```python
from build123d import *

# Parameters (mm, degrees)
F0_R      = 14.3002
F1_DEPTH  = 40.5892
F2_W      = 11.867738
F2_H      = 43.622876
F2_W_2    = 10.350018
F3_DEPTH  = 37.084
F5_R      = 18.288
F6_DEPTH  = 1.651
F7_W      = 12.7
F7_H      = 5.3975
F8_DEPTH  = 9.7536
F9_W      = 0.7874
F9_H      = 7.62
F9_W_2    = 0.8128
F10_DEPTH = 9.5631


with BuildPart() as f1:
    # F0 (on Front) → F1 (new body)
    with BuildSketch(Plane.XZ):
        Circle(F0_R)
    extrude(amount=-F1_DEPTH)

    # F2 (on face) → F3 (cut)
    with BuildSketch(Plane.XZ):
        with Locations((-19.027569, 0.496973)):
            Rectangle(F2_W, F2_H)
        with Locations((18.268709, 0.496973)):
            Rectangle(F2_W_2, F2_H)
    extrude(amount=-F3_DEPTH, mode=Mode.SUBTRACT)

    # F5 (on offset) → F6 (join)
    with BuildSketch(Plane(origin=(0, 38.6842, 0), x_dir=(1, 0, 0), z_dir=(0, 1, 0))):
        Circle(F5_R)
    extrude(amount=-F6_DEPTH)

    # F7 (on face) → F8 (cut)
    with BuildSketch(Plane(origin=(0, 40.5892, 0), x_dir=(-1, 0, 0), z_dir=(0, 1, 0))):
        with Locations((0, 4.15925)):
            Rectangle(F7_W, F7_H)
        with Locations((0, -4.15925)):
            Rectangle(F7_W, F7_H)
    extrude(amount=-F8_DEPTH, mode=Mode.SUBTRACT)

    # F9 (on face) → F10 (join)
    with BuildSketch(Plane.XZ):
        with Locations((-4.572, -0.381)):
            Rectangle(F9_W, F9_H)
        with Locations((5.5499, -0.381)):
            Rectangle(F9_W_2, F9_H)
    extrude(amount=F10_DEPTH)


solid = f1.part
```
The model under review builds one solid part; all positions refer to its coordinate system, in mm. A direction names the side the tool comes from. Round coordinates to 2 decimals unless told otherwise and drop trailing zeros. Order: outer loops, then holes, each group sorted by start corner. A loop starts at its lowest first (then second) coordinate and runs counter-clockwise, first axis right, second up.
Item 1: Add section C-C, the plane y = 19.5. State the section outline as (x, z) points.
Working result:
outline: (-13.09, -5.75) arc R14.3 ccw to (13.09, -5.75) - (13.09, 5.75) arc R14.3 ccw to (-13.09, 5.75) - close
Item 2: Machinability: for faces 1 (the flat face through (5.956, -5, 0)), 2 (the flat face through (6.35, 36, 4)), 3 (the flat face through (-13.094, 18, 0)), which of the approach directions +Z, -Z, +X, -X, +Y, -Y give a long, thin tool a straight path to every point of the face, cutting with its end or side? Answer none if there is none.
Working result:
face 1: +Z, -Z, +X, -Y
face 2: +Y
face 3: +Z, -Z, -X, -Y
Item 3: For pin 1 (5 mm diameter, centred on y = 35.5, z = 3, fed in from -X); pin 2 (3 mm diameter, centred on x = -2.5, z = -6.5, fed in from -Y); pin 3 (10 mm diameter, centred on x = 12, y = 20.5, fed in from -Z), all flat-tipped, find the tip position at first contact; note any pin that passes through.
Working result:
pin 1: stops at x = -18.26
pin 2: stops at y = 0
pin 3: stops at z = -12.47
Item 4: To check wall thickness, follow probe 1 along Z at (x, y) = (5, 32); probe 2 along Z at (x, y) = (-3.5, 37); probe 3 along X at (y, z) = (-3.5, 1). State the ranges of each line that lie inside material, in increasing order.
Working result:
probe 1: z = -13.4 to -6.86, -1.46 to 1.46, 6.86 to 13.4
probe 2: z = -13.87 to -6.86, -1.46 to 1.46, 6.86 to 13.87
probe 3: x = -4.97 to -4.18, 5.14 to 5.96
Item 5: Add section B-B, the plane z = 0. State the section outline as (x, y) points, and give its area (3 significant figures).
Working result:
outline: (-18.29, 37.03) - (-13.09, 37.03) - (-13.09, 0) - (-4.97, 0) - (-4.97, -9.56) - (-4.18, -9.56) - (-4.18, 0) - (5.14, 0) - (5.14, -9.56) - (5.96, -9.56) - (5.96, 0) - (13.09, 0) - (13.09, 37.03) - (18.29, 37.03) - (18.29, 38.68) - (14.3, 38.68) - (14.3, 40.59) - (-14.3, 40.59) - (-14.3, 38.68) - (-18.29, 38.68) - close
area: 1,100 mm2
Item 6: Add section A-A, the plane x = 0. State the section outline as (y, z) points.
Working result:
outline: (0, -14.3) - (37.03, -14.3) - (37.03, -18.29) - (38.68, -18.29) - (38.68, -14.3) - (40.59, -14.3) - (40.59, -6.86) - (30.84, -6.86) - (30.84, -1.46) - (40.59, -1.46) - (40.59, 1.46) - (30.84, 1.46) - (30.84, 6.86) - (40.59, 6.86) - (40.59, 14.3) - (38.68, 14.3) - (38.68, 18.29) - (37.03, 18.29) - (37.03, 14.3) - (0, 14.3) - close
Item 7: Add section D-D, the plane x = 10. State the section outline as (y, z) points.
Working result:
outline: (0, -10.22) - (37.03, -10.22) - (37.03, -15.31) - (38.68, -15.31) - (38.68, -10.22) - (40.59, -10.22) - (40.59, 10.22) - (38.68, 10.22) - (38.68, 15.31) - (37.03, 15.31) - (37.03, 10.22) - (0, 10.22) - close
